Build history of the part. All positions in model axes, mm. A direction names the side the tool comes from. Round coordinates to 2 decimals unless told otherwise and drop trailing zeros. Order: outer loops, then holes, each group sorted by start corner. A loop starts at its lowest first (then second) coordinate and runs counter-clockwise, first axis right, second up. Notation, with made-up numbers: M -32,35 L -5,35 A23 cw -5,71 Z; hole C 65.25,53.5 d10. An arc over 180 degrees is marked long. Use CSV: the item, a comma, the result in double quotes.
from build123d import *

# Parameters (mm, degrees)
SKETCH_1_R          = 13.1
EXTRUDE_1_DEPTH     = 11.8
SKETCH_3_R          = 1.5
CUT_EXTRUDE_1_DEPTH = 5
SKETCH_4_R          = 1.5
CUT_EXTRUDE_2_DEPTH = 15


with BuildPart() as part:
    # 草图1 → 凸台-拉伸1 (new body)
    with BuildSketch(Plane.XY):
        Circle(SKETCH_1_R)
    extrude(amount=EXTRUDE_1_DEPTH)

    # 草图3 → 切除-拉伸1 (cut)
    with BuildSketch(Plane.XY.offset(11.8)):
        with Locations((-9.75, 0)):
            Circle(SKETCH_3_R)
        with Locations((0, 9.75)):
            Circle(SKETCH_3_R)
        with Locations((9.75, 0)):
            Circle(SKETCH_3_R)
        with Locations((0, -9.75)):
            Circle(SKETCH_3_R)
    extrude(amount=-CUT_EXTRUDE_1_DEPTH, mode=Mode.SUBTRACT)

    # 草图4 → 切除-拉伸2 (cut)
    with BuildSketch(Plane.XY.offset(11.8)):
        with Locations((-9.75, 0)):
            Circle(SKETCH_4_R)
        with Locations((9.75, 0)):
            Circle(SKETCH_4_R)
        with BuildLine():
            Line((-5.5, -1.5), (-5.5, 1.5))
            Line((-5.5, 1.5), (-3.708099244, 1.5))
            ThreePointArc((-3.708099244, 1.5), (4, 0), (-3.708099244, -1.5))
            Line((-3.708099244, -1.5), (-5.5, -1.5))
        make_face()
    extrude(amount=-CUT_EXTRUDE_2_DEPTH, mode=Mode.SUBTRACT)


solid = part.part
(1) Wall check: line 1 (Y direction, x = 0, z = 9); line 2 (Z direction, x = 0.5, y = 10.25); line 3 (X direction, y = 8.5, z = 10). Give the ranges that are in metal, low to high. Write a range as from..to.
Answer block:
line 1,"y = -13.1..-11.25, -8.25..-4, 4..8.25, 11.25..13.1"
line 2,"z = 0..6.8"
line 3,"x = -9.97..-0.83, 0.83..9.97"
(2) Cut at B-B, the plane x = 0. Give the cut face in (y, z), and give its area (3 significant figures).
Answer block:
outline,"M -13.1,0 L -4,0 L -4,11.8 L -8.25,11.8 L -8.25,6.8 L -11.25,6.8 L -11.25,11.8 L -13.1,11.8 Z; M 4,0 L 13.1,0 L 13.1,11.8 L 11.25,11.8 L 11.25,6.8 L 8.25,6.8 L 8.25,11.8 L 4,11.8 Z"
area,"185 mm²"
(3) Cut at D-D, the plane z = 6.25. Give the cut face in (x, y), and give its area (3 significant figures).
Answer block:
outline,"C 0,0 d26.2; hole C -9.75,0 d3; hole M -5.5,-1.5 L -3.71,-1.5 A4 ccw long -3.71,1.5 L -5.5,1.5 Z; hole C 9.75,0 d3"
area,"470 mm²"
(4) Two-plate mould, pull along Y, no slides. Class faces 4 (the face through (-0.325, -11.214, 9.335)), 5 (the face through (3, 3, 0)), 6 (the face through (-1.705, 12.989, 5.817)): released by +Y, released by -Y, zero draft, split by the parting line, or undercut.
Answer block:
face 4,"undercut"
face 5,"zero draft"
face 6,"split by the parting line"
(5) Cut at A-A, the plane y = 0. Give the cut face in (x, z), and give its area (3 significant figures).
Answer block:
outline,"M -13.1,0 L -11.25,0 L -11.25,11.8 L -13.1,11.8 Z; M -8.25,0 L -5.5,0 L -5.5,11.8 L -8.25,11.8 Z; M 4,0 L 8.25,0 L 8.25,11.8 L 4,11.8 Z; M 11.25,0 L 13.1,0 L 13.1,11.8 L 11.25,11.8 Z"
area,"126 mm²"
(6) Cut at C-C, the plane z = 10. Give the cut face in (x, y).
Answer block:
outline,"C 0,0 d26.2; hole C -9.75,0 d3; hole M -5.5,-1.5 L -3.71,-1.5 A4 ccw long -3.71,1.5 L -5.5,1.5 Z; hole C 0,-9.75 d3; hole C 0,9.75 d3; hole C 9.75,0 d3"
(7) Tool access for faces 1 (the face through (3, 3, 11.8)), 2 (the face through (-5.5, 0, 6)), 3 (the face through (-0.325, 8.286, 9.335)): list every direction of +Z, -Z, +X, -X, +Y, -Y with a clear straight run to the whole face (end or side of a thin tool).
Answer block:
face 1,"+Z, +X, -X, +Y, -Y"
face 2,"+Z, -Z"
face 3,"+Z"
(8) Drop flat-ended pins along their axis: pin 1 (3 mm diameter, centred on y = 6, z = 6, fed in from -X); pin 2 (8 mm diameter, centred on x = -5, y = 8.5, fed in from -Z); pin 3 (2 mm diameter, centred on x = -4.5, z = 7.5, fed in from +Y); pin 4 (1.8 mm diameter, centred on x = 0, y = -9.75, fed in from +Z). Give the stop position or say it passes through.
Answer block:
pin 1,"stops at x = -12.3"
pin 2,"stops at z = 0"
pin 3,"stops at y = 12.62"
pin 4,"stops at z = 6.8"
